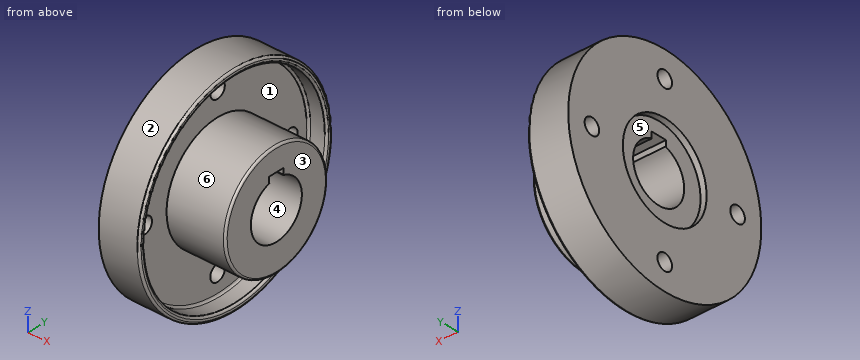
from build123d import *

# Parameters (mm, degrees)
SKETCH2_R          = 28
CUT_EXTRUDE1_DEPTH = 170.917627102
SKETCH3_R          = 46
CUT_EXTRUDE2_DEPTH = 6
SKETCH4_W          = 6
SKETCH4_H          = 16
CUT_EXTRUDE6_DEPTH = 168.176553424
SKETCH5_R          = 8
CUT_EXTRUDE7_DEPTH = 170.917627149
CIRPATTERN1_COUNT  = 4


with BuildPart() as part:
    # Sketch1 → Revolve1 (revolve)
    with BuildSketch(Plane.XY, mode=Mode.PRIVATE) as revolve1_sk:
        with BuildLine():
            Line((0, 0), (80, 0))
            Line((80, 0), (80, 54))
            ThreePointArc((80, 54), (79.414213562, 55.414213562), (78, 56))
            Line((78, 56), (28.292682927, 56))
            Line((28.292682927, 56), (22, 56))
            Line((22, 56), (22, 98))
            ThreePointArc((22, 98), (22.585786438, 99.414213562), (24, 100))
            Line((24, 100), (38, 100))
            ThreePointArc((38, 100), (39.414213562, 100.585786438), (40, 102))
            Line((40, 102), (40, 104))
            ThreePointArc((40, 104), (39.414213562, 105.414213562), (38, 106))
            Line((38, 106), (0, 106))
            Line((0, 106), (0, 0))
        make_face()
    revolve(revolve1_sk.sketch.rotate(Axis((0, 0, 0), (1, 0, 0)), 90), axis=Axis((0, 0, 0), (1, 0, 0)))

    # Sketch2 → Cut-Extrude1 (cut, through all)
    with BuildSketch(Plane(origin=(80, 0, 0), x_dir=(0, 0, -1), z_dir=(1, 0, 0))):
        Circle(SKETCH2_R)
    extrude(amount=-CUT_EXTRUDE1_DEPTH, mode=Mode.SUBTRACT)

    # Sketch3 → Cut-Extrude2 (cut)
    with BuildSketch(Plane.ZY):
        Circle(SKETCH3_R)
    extrude(amount=-CUT_EXTRUDE2_DEPTH, mode=Mode.SUBTRACT)

    # Sketch4 → Cut-Extrude6 (cut, through all)
    with BuildSketch(Plane.ZY.offset(-6)):
        with Locations((30, 0)):
            Rectangle(SKETCH4_W, SKETCH4_H)
    extrude(amount=-CUT_EXTRUDE6_DEPTH, mode=Mode.SUBTRACT)

    # Sketch5 → Cut-Extrude7 (cut, through all)
    with BuildSketch(Plane.ZY):
        with Locations((0, 80)):
            Circle(SKETCH5_R)
    cut_extrude7 = extrude(amount=-CUT_EXTRUDE7_DEPTH, mode=Mode.SUBTRACT)

    # CirPattern1: Cut-Extrude7 ×4 about axis
    cirpattern1_axis = Axis((0, 0, 0), (1, 0, 0))
    for i in range(1, CIRPATTERN1_COUNT):
        add(cut_extrude7.rotate(cirpattern1_axis, i * 360 / CIRPATTERN1_COUNT), mode=Mode.SUBTRACT)


solid = part.part
Geometry: final body of the model. Coordinates: model frame, mm. Face numbers are marked on the shaded views. A direction names the side the tool comes from. Give positions to 0.01 mm unless a question says otherwise; leave off trailing zeros. Loops run counter-clockwise (first coordinate to the right, second up) from the corner with the lowest first, then second, coordinate; pieces in that order, holes last. Notation, with made-up numbers: (32, 42) -> (90, 42) arc R22 ccw to (90, 78) -> close; hole circle Ø7 at (29.5, -40). An arc over 180 degrees is marked (long way). Put each result on its own line as item: value.
1. Cut plane B-B (x = 43.5). Return the cut outline in (y, z), plus the area to 3 significant figures.
Taken from the geometry:
outline: circle Ø112 at (0, 0); hole (-8, 27) -> (-7.42, 27) arc R28 ccw (long way) to (7.42, 27) -> (8, 27) -> (8, 33) -> (-8, 33) -> close
area: 7,300 mm2
2. Cut plane C-C (y = 0). Count the separate pieces of the cut face and the enclosed holes in it, plus the area to 3 significant figures.
Taken from the geometry:
separate pieces: 4
enclosed holes: 0
area: 5,600 mm2
3. Cut plane A-A (x = 29). Return the cut outline in (y, z).
Taken from the geometry:
outline: circle Ø212 at (0, 0); circle Ø112 at (0, 0); hole circle Ø200 at (0, 0); hole (-8, 27) -> (-7.42, 27) arc R28 ccw (long way) to (7.42, 27) -> (8, 27) -> (8, 33) -> (-8, 33) -> close
4. Ray query, line 1 along Y through (x, z) = (12.25, 0); line 2 along Y through (x, z) = (3, 0); line 3 along Z through (x, y) = (13.5, -1.5). Return the intervals inside material, ascending. Write a range as [from, to].
Taken from the geometry:
line 1: y = [-106, -88], [-72, -28], [28, 72], [88, 106]
line 2: y = [-106, -88], [-72, -46], [46, 72], [88, 106]
line 3: z = [-105.99, -87.86], [-72.14, -27.96], [33, 72.14], [87.86, 105.99]
5. Set-up query: the marked faces 4, 5 and 6. Return all of +Z, -Z, +X, -X, +Y, -Y with unobstructed straight access to the full face (end or side cutting, diameter ignored); none if empty.
Taken from the geometry:
face 4: +X, -X
face 5: -X
face 6: +X
6. Pin query (flat end, axial travel): P1, Ø21, axis at y = 80, z = 0, coming from the +X side; P2, Ø5, axis at x = 48.5, z = 31, coming from the -Y side; P3, Ø14.5, axis at y = 0, z = 80, coming from the +X side; P4, Ø0.5, axis at x = 49.5, y = -8, coming from the +Z side. Return the tip coordinate at first contact, or that it passes through.
Taken from the geometry:
P1: stops at x = 22
P2: stops at y = -48.21
P3: passes through
P4: stops at z = 55.46
7. Pull-direction query (Z, two-part tool) for the marked faces 1, 2 and 3; classes: released by +Z, released by -Z, zero draft, split by the parting line, or undercut.
Taken from the geometry:
face 1: undercut
face 2: split by the parting line
face 3: zero draft
